from build123d import *

# Parameters (mm, degrees)
SZKIC1_W                    = 75
SZKIC1_H                    = 13
SZKIC2_R                    = 32
DODANIE_WYCI_GNI_CIE1_DEPTH = 19
DODANIE_WYCI_GNI_CIE1_TAPER = 22.448353305
SZKIC3_R                    = 24.15
DODANIE_WYCI_GNI_CIE2_DEPTH = 7
SZKIC4_R                    = 47
DODANIE_WYCI_GNI_CIE3_DEPTH = 3
DODANIE_WYCI_GNI_CIE3_TAPER = 45
OTW_R_18_0_18_1_D           = 18
OTW_R_18_0_18_1_DEPTH       = 13
OTW_R_POD_RUB_M391_D        = 43.1
ZAOKR_GLENIE1_R             = 6


with BuildPart() as part:
    # Szkic1 → Obrót1 (revolve)
    with BuildSketch(Plane(origin=(0, 0, 0), x_dir=(-1, 0, 0), z_dir=(0, 0, -1)), mode=Mode.PRIVATE) as obr_t1_sk:
        with Locations((-37.5, 9.5)):
            Rectangle(SZKIC1_W, SZKIC1_H)
    revolve(obr_t1_sk.sketch.rotate(Axis((0, 3, 0), (0, 1, 0)), 270), axis=Axis((0, 3, 0), (0, 1, 0)))

    # Szkic2 → Dodanie-wyciągnięcie1 (add)
    with BuildSketch(Plane(origin=(0, 16, 0), x_dir=(-1, 0, 0), z_dir=(0, 1, 0))):
        Circle(SZKIC2_R)
    extrude(amount=DODANIE_WYCI_GNI_CIE1_DEPTH, taper=DODANIE_WYCI_GNI_CIE1_TAPER)

    # Szkic3 → Dodanie-wyciągnięcie2 (add)
    with BuildSketch(Plane(origin=(0, 35, 0), x_dir=(-1, 0, 0), z_dir=(0, 1, 0))):
        with Locations(Location((0, 0, 0), (0, 0, 270))):
            Circle(SZKIC3_R)
    extrude(amount=DODANIE_WYCI_GNI_CIE2_DEPTH)

    # Szkic4 → Dodanie-wyciągnięcie3 (add)
    with BuildSketch(Plane.XZ.offset(-3)):
        Circle(SZKIC4_R)
    extrude(amount=DODANIE_WYCI_GNI_CIE3_DEPTH, taper=DODANIE_WYCI_GNI_CIE3_TAPER)

    # Otwór Ø18.0 (18)1
    with Locations(Plane(origin=(0, 16, 0), x_dir=(1, 0, 0), z_dir=(0, 1, 0))):
        with Locations((-55, 0), (55, 0), (0, -55), (0, 55)):
            Hole(OTW_R_18_0_18_1_D / 2, depth=OTW_R_18_0_18_1_DEPTH)

    # Otwór pod śrubę M391 (through all)
    with Locations(Plane(origin=(0, 42, 0), x_dir=(1, 0, 0), z_dir=(0, 1, 0))):
        with Locations((0, 0)):
            Hole(OTW_R_POD_RUB_M391_D / 2)

    # Zaokrąglenie1
    zaokr_glenie1_edges = [part.edges().sort_by_distance(p)[0] for p in [
        (32, 16, 0),
    ]]
    fillet(zaokr_glenie1_edges, radius=ZAOKR_GLENIE1_R)


solid = part.part
Verification items for the finished model (mm, model axes). A direction names the side the tool comes from. Round coordinates to 2 decimals unless told otherwise and drop trailing zeros. Loops run counter-clockwise (first coordinate to the right, second up) from the corner with the lowest first, then second, coordinate; pieces in that order, holes last. Notation, with made-up numbers: (-13, 5.5) - (21, 5.5) arc R31 cw to (21, 33.5) - close; hole circle Ø9 at (10, -36). An arc over 180 degrees is marked (long way). Write item = value, one per line.
Q1. Material ranges on L1, parallel to Z at x = -5.5, y = 6; L2, parallel to Y at x = 17, z = -33.5; L3, parallel to Z at x = 10, y = 38, recorded low to high.
Here are the results:
L1 = -74.8 to -62.12, -47.88 to -20.84, 20.84 to 47.88, 62.12 to 74.8
L2 = 0 to 16
L3 = -21.98 to -19.09, 19.09 to 21.98
Q2. Sectioned sample at A-A on y = 6. Record the boundary of the cut face in (x, z), plus the area to 3 significant figures.
Here are the results:
outline = circle Ø150 at (0, 0); hole circle Ø18 at (-55, 0); hole circle Ø43.1 at (0, 0); hole circle Ø18 at (0, -55); hole circle Ø18 at (0, 55); hole circle Ø18 at (55, 0)
area = 15,200 mm^2
Q3. Sectioned sample at D-D on x = 55. Record the boundary of the cut face in (y, z).
Here are the results:
outline = (3, -50.99) - (16, -50.99) - (16, -9) - (3, -9) - close; (3, 9) - (16, 9) - (16, 50.99) - (3, 50.99) - close
Q4. Depth check by flat-ended pin: pin 1 (3 mm diameter, centred on x = 6, z = 19, fed in from +Y); pin 2 (3 mm diameter, centred on x = 55.5, y = 16.5, fed in from -Z); pin 3 (0.5 mm diameter, centred on x = 0.5, z = -46.5, fed in from +Y); pin 4 (1.1 mm diameter, centred on x = -46.5, z = 0, fed in from +Y). Enter the tip coordinate at first touch or a pass-through.
Here are the results:
pin_1 = through
pin_2 = -51.96
pin_3 = 3
pin_4 = 16
Q5. Sectioned sample at C-C on z = 0. State how many separate pieces and enclosed holes the cut face has, plus the area to 3 significant figures.
Here are the results:
separate_pieces = 4
enclosed_holes = 0
area = 1,360 mm^2
Q6. Tool access check on faces 5 (the cylindrical face through (-45.636, 9.591, -59.517)), 6 (the flat face through (-32.3, 3, -34.4)), 7 (the cylindrical face through (46.416, 9.409, -2.703)). Record the directions out of +Z, -Z, +X, -X, +Y, -Y that give a thin tool (end or side, any length) a straight path to the whole face; none if there is none.
Here are the results:
face_5 = +Y, -Y
face_6 = -Y
face_7 = +Y
Q7. Mould release check, pull along Z, two halves, no side actions. Record for faces 1 (the cylindrical face through (-4.84, 9.41, -62.59)), 2 (the cylindrical face through (-20.555, 20.706, -6.473)), 3 (the cylindrical face through (-7.254, 38.451, -23.035)), 4 (the flat face through (0, 42, 22)): +Z half, -Z half, draft (parallel to the pull), parting line (faces both ways), or undercut.
Here are the results:
face_1 = undercut
face_2 = undercut
face_3 = parting line
face_4 = draft
Q8. Sectioned sample at B-B on x = 0. Record the boundary of the cut face in (y, z), plus the area to 3 significant figures.
Here are the results:
outline = (0, -44) - (3, -47) - (3, -46) - (16, -46) - (16, -36.01) arc R6 cw to (19.71, -30.47) - (35, -24.15) - (42, -24.15) - (42, -21.55) - (0, -21.55) - close; (0, 21.55) - (42, 21.55) - (42, 24.15) - (35, 24.15) - (19.71, 30.47) arc R6 cw to (16, 36.01) - (16, 46) - (3, 46) - (3, 47) - (0, 44) - close; (3, -75) - (16, -75) - (16, -64) - (3, -64) - close; (3, 64) - (16, 64) - (16, 75) - (3, 75) - close
area = 1,360 mm^2
